```python
from build123d import *

# Parameters (mm, degrees)
BOSS_EXTRUDE1_DEPTH             = 12.7
BOSS_EXTRUDE4_REACH             = 14.7
BOSS_EXTRUDE4_DIRECTION_2_REACH = 14.7
SKETCH6_W                       = 16.51
SKETCH6_H                       = 15.748
CUT_EXTRUDE2_DEPTH              = 61.96
SKETCH11_W                      = 20.32
SKETCH11_H                      = 7.62
CUT_EXTRUDE3_DEPTH              = 3.81
SKETCH15_R                      = 3.2385
CUT_EXTRUDE4_DEPTH              = 25.4
SKETCH16_W                      = 16.51
SKETCH16_H                      = 12.7
CUT_EXTRUDE5_DEPTH              = 36.83


with BuildPart() as part:
    # Sketch1 → Boss-Extrude1 (new body, symmetric)
    with BuildSketch(Plane.XY):
        with BuildLine():
            Line((-20.32, 16.002), (-20.32, -38.1))
            Line((-20.32, -38.1), (20.32, -38.1))
            Line((20.32, -38.1), (20.32, 16.002))
            Line((20.32, 16.002), (2.794, 16.002))
            Line((2.794, 16.002), (2.794, 28.1305))
            Line((2.794, 28.1305), (6.477, 28.1305))
            ThreePointArc((6.477, 28.1305), (6.946330803, 28.444096816), (6.836210245, 28.997710245))
            Line((6.836210245, 28.997710245), (3.706459265, 32.127461224))
            ThreePointArc((3.706459265, 32.127461224), (2.882423959, 32.678064013), (1.910408041, 32.87141))
            Line((1.910408041, 32.87141), (-1.910408041, 32.87141))
            ThreePointArc((-1.910408041, 32.87141), (-2.882423959, 32.678064013), (-3.706459265, 32.127461224))
            Line((-3.706459265, 32.127461224), (-6.836210245, 28.997710245))
            ThreePointArc((-6.836210245, 28.997710245), (-6.946330803, 28.444096816), (-6.477, 28.1305))
            Line((-6.477, 28.1305), (-2.794, 28.1305))
            Line((-2.794, 28.1305), (-2.794, 16.002))
            Line((-2.794, 16.002), (-20.32, 16.002))
        make_face()
        Polygon((-4.106115114, 7.112), (-8.212230229, 0), (-4.106115114, -7.112), (4.106115114, -7.112), (8.212230229, 0), (4.106115114, 7.112), align=None, mode=Mode.SUBTRACT)
    extrude(amount=BOSS_EXTRUDE1_DEPTH, both=True)

    # Boss-Extrude4: up to this face of the body (flat: up to its plane)
    boss_extrude4_end = Plane(part.part.faces().sort_by_distance((0, -9.949298675, 12.7))[0])
    # Sketch10 → Boss-Extrude4 (add, up to the picked face)
    with BuildSketch(Plane.XY, mode=Mode.PRIVATE) as boss_extrude4_sk1:
        Polygon((-20.32, -38.1), (-20.32, -53.34), (-40.64, -53.34), (-40.64, -57.15), (-16.51, -57.15), (-16.51, -38.1), align=None)
    boss_extrude4_tool1 = split(extrude(boss_extrude4_sk1.sketch, amount=BOSS_EXTRUDE4_REACH, mode=Mode.PRIVATE), bisect_by=boss_extrude4_end, keep=Keep.BOTH, mode=Mode.PRIVATE)
    add(boss_extrude4_tool1.solids().sort_by_distance((-20.012566, -45.72, 0))[0])

    # Boss-Extrude4 direction 2: up to this face of the body (flat: up to its plane)
    boss_extrude4_direction_2_end = Plane(part.part.faces().sort_by_distance((0, -9.949298675, -12.7))[0])
    # Sketch10 → Boss-Extrude4 direction 2 (add, up to the picked face)
    with BuildSketch(Plane.XY, mode=Mode.PRIVATE) as boss_extrude4_direction_2_sk1:
        Polygon((-20.32, -38.1), (-20.32, -53.34), (-40.64, -53.34), (-40.64, -57.15), (-16.51, -57.15), (-16.51, -38.1), align=None)
    boss_extrude4_direction_2_tool1 = split(extrude(boss_extrude4_direction_2_sk1.sketch, amount=-BOSS_EXTRUDE4_DIRECTION_2_REACH, mode=Mode.PRIVATE), bisect_by=boss_extrude4_direction_2_end, keep=Keep.BOTH, mode=Mode.PRIVATE)
    add(boss_extrude4_direction_2_tool1.solids().sort_by_distance((-20.012566, -45.72, 0))[0])

    # Sketch6 → Cut-Extrude2 (cut, through all)
    with BuildSketch(Plane(origin=(20.32, 0, 0), x_dir=(0, 0, -1), z_dir=(1, 0, 0))):
        with Locations((0, -17.526)):
            Rectangle(SKETCH6_W, SKETCH6_H)
    extrude(amount=-CUT_EXTRUDE2_DEPTH, mode=Mode.SUBTRACT)

    # Sketch11 → Cut-Extrude3 (cut)
    with BuildSketch(Plane(origin=(0, -53.34, 0), x_dir=(1, 0, 0), z_dir=(0, 1, 0))):
        with Locations((-30.48, 0)):
            Rectangle(SKETCH11_W, SKETCH11_H)
    extrude(amount=-CUT_EXTRUDE3_DEPTH, mode=Mode.SUBTRACT)

    # Sketch15 → Cut-Extrude4 (cut)
    with BuildSketch(Plane.XY.offset(12.7)):
        with Locations((0, -19.05)):
            Circle(SKETCH15_R)
    extrude(amount=-CUT_EXTRUDE4_DEPTH, mode=Mode.SUBTRACT)

    # Sketch16 → Cut-Extrude5 (cut)
    with BuildSketch(Plane(origin=(20.32, 0, 0), x_dir=(0, 0, -1), z_dir=(1, 0, 0))):
        with Locations((0, -31.75)):
            Rectangle(SKETCH16_W, SKETCH16_H)
    extrude(amount=-CUT_EXTRUDE5_DEPTH, mode=Mode.SUBTRACT)


solid = part.part
```
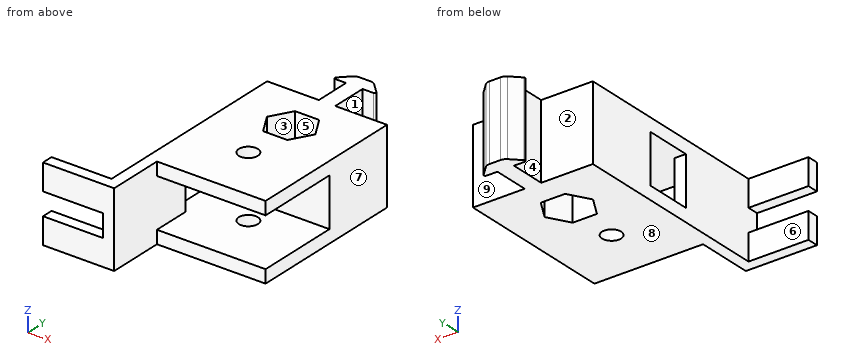
Geometry: final body of the model. Coordinates: model frame, mm. Face numbers are marked on the shaded views. A direction names the side the tool comes from. Coordinates: 2 decimals unless noted, no trailing zeros. Order: outer loops, then holes, each group sorted by start corner. A loop starts at its lowest first (then second) coordinate and runs counter-clockwise, first axis right, second up. Notation, with made-up numbers: M 2,29.25 L 57,29.25 A34 cw 57,68.25 Z; hole C 80.5,18 d4. An arc over 180 degrees is marked long. Answer as CSV lines item,"result".
Q1. First-contact query: P1, Ø13.5, axis at y = 23.5, z = 2, coming from the +X side (3 decimals); P2, Ø1.9, axis at x = -18, z = -3, coming from the +Y side; P3, Ø2.5, axis at x = -28, z = 7.5, coming from the +Y side; P4, Ø5, axis at x = 0, y = -19.05, coming from the -Z side. Flat tips, straight axial feed; report the tip coordinate or a pass-through.
Answers:
P1,"stops at x = 6.985"
P2,"stops at y = 16"
P3,"stops at y = -53.34"
P4,"passes through"
Q2. Section D-D on x = 0. Return the cut outline in (y, z) (1 decimal), and give its area (3 significant figures).
Answers:
outline,"M -38.1,-12.7 L -22.3,-12.7 L -22.3,-8.3 L -38.1,-8.3 Z; M -38.1,8.3 L -22.3,8.3 L -22.3,12.7 L -38.1,12.7 Z; M -15.8,-12.7 L -7.1,-12.7 L -7.1,12.7 L -15.8,12.7 L -15.8,8.3 L -9.7,8.3 L -9.7,-8.3 L -15.8,-8.3 Z; M 7.1,-12.7 L 32.9,-12.7 L 32.9,12.7 L 7.1,12.7 Z"
area,"914 mm^2"
Q3. Section A-A on z = -7. Return the cut outline in (x, y).
Answers:
outline,"M -40.64,-57.15 L -16.51,-57.15 L -16.51,-25.4 L -20.32,-25.4 L -20.32,-53.34 L -40.64,-53.34 Z; M -20.32,-9.65 L 20.32,-9.65 L 20.32,16 L 2.79,16 L 2.79,28.13 L 6.48,28.13 A0.51 ccw 6.84,29 L 3.71,32.13 A2.54 ccw 1.91,32.87 L -1.91,32.87 A2.54 ccw -3.71,32.13 L -6.84,29 A0.51 ccw -6.48,28.13 L -2.79,28.13 L -2.79,16 L -20.32,16 Z; hole M -8.21,0 L -4.11,-7.11 L 4.11,-7.11 L 8.21,0 L 4.11,7.11 L -4.11,7.11 Z"
Q4. Section B-B on x = -30. Return the cut outline in (y, z).
Answers:
outline,"M -57.15,-12.7 L -53.34,-12.7 L -53.34,-3.81 L -57.15,-3.81 Z; M -57.15,3.81 L -53.34,3.81 L -53.34,12.7 L -57.15,12.7 Z"
Q5. Draft query along X for the marked faces 1, 2, 3 and 4. Return one class per face: pulls with the +X half, pulls with the -X half, needs draft (parallel to the pull), parting line crosses it, or undercut.
Answers:
face 1,"pulls with the +X half"
face 2,"needs draft"
face 3,"undercut"
face 4,"pulls with the -X half"
Q6. Set-up query: the marked faces 5, 6, 7, 8 and 9. Return all of +Z, -Z, +X, -X, +Y, -Y with unobstructed straight access to the full face (end or side cutting, diameter ignored); none if empty.
Answers:
face 5,"+Z, -Z"
face 6,"+Z, -Z, -X, +Y"
face 7,"+Z, -Z, +X, +Y, -Y"
face 8,"-Z, +X, -X, +Y, -Y"
face 9,"+Z, -Z, +X"
Q7. Line query: probe 1 along Y at (x, z) = (0, 9.7); probe 2 along Z at (x, y) = (-13, -14) (3 decimals); probe 3 along Y at (x, z) = (1.5, 3). Output: solid intervals per line, ascending. Write a range as [from, to].
Answers:
probe 1,"y = [-38.1, -22.29], [-15.81, -7.11], [7.11, 32.87]"
probe 2,"z = [-12.7, -8.255], [8.255, 12.7]"
probe 3,"y = [-9.65, -7.11], [7.11, 32.87]"
Q8. Section C-C on y = -19.05. Return the cut outline in (x, z) (1 decimal), and give its area (3 significant figures).
Answers:
outline,"M -20.3,-12.7 L -3.2,-12.7 L -3.2,-8.3 L -20.3,-8.3 Z; M -20.3,8.3 L -3.2,8.3 L -3.2,12.7 L -20.3,12.7 Z; M 3.2,-12.7 L 20.3,-12.7 L 20.3,-8.3 L 3.2,-8.3 Z; M 3.2,8.3 L 20.3,8.3 L 20.3,12.7 L 3.2,12.7 Z"
area,"304 mm^2"
